Check sheet for the modelled part. Datum: model origin and axes. Units: mm. A direction names the side the tool comes from. Round coordinates to 2 decimals unless told otherwise and drop trailing zeros. Order: outer loops, then holes, each group sorted by start corner. A loop starts at its lowest first (then second) coordinate and runs counter-clockwise, first axis right, second up.
Q1. Depth check by flat-ended pin: P1, Ø3.5, axis at y = 25, z = 10.5, coming from the -X side; P2, Ø0.9, axis at x = 17, y = 19, coming from the -Z side; P3, Ø6, axis at y = 23, z = 10.5, coming from the +X side. Enter the tip coordinate at first touch or a pass-through.
Q2. Cross-section at A-A on x = 2. Record the cut outline in (y, z), then the cut area to 3 significant figures.
Q3. Set-up check for faces 1 (the flat face through (2.935, 17, 16)), 2 (the cylindrical face through (12.252, 20.541, 9.077)), 3 (the flat face through (16, 17, 17.161)), 4 (the flat face through (16.435, 17, 9)), 5 (the flat face through (1.435, 17, 9)): record each of +Z, -Z, +X, -X, +Y, -Y from which the full face is reachable in a straight line by a thin tool's end or side.
Q4. Cross-section at C-C on y = 6.5. Record the cut outline in (x, z).
Q5. Scan lines: probe 1 along Y at (x, z) = (9, 12); probe 2 along Z at (x, y) = (2, 2); probe 3 along Z at (x, y) = (5.25, 18.5). Record each from-to range of solid material in increasing order.
Q6. Cross-section at B-B on z = 11.25. Record the cut outline in (x, y).
Q7. Mould release check, pull along X, two halves, no side actions. Record for faces 6 (the flat face through (-0.065, 17, 18)), 7 (the flat face through (16, 17, 15.161)), 8 (the flat face through (9, 18, 15.161)): +X half, -X half, draft (parallel to the pull), parting line (faces both ways), or undercut.
Q8. Cross-section at D-D on x = 17. Record the cut outline in (y, z), then the cut area to 3 significant figures.
from build123d import *

# Parameters (mm, degrees)
SKETCH1_W           = 6
SKETCH1_H           = 2
BOSS_EXTRUDE1_DEPTH = 35
SKETCH2_R           = 4.5
CUT_EXTRUDE1_DEPTH  = 12


with BuildPart() as part:
    # Sketch1 → Boss-Extrude1 (new body)
    with BuildSketch(Plane(origin=(0, 0, 0), x_dir=(1, 0, 0), z_dir=(0, 1, 0))):
        Polygon((1.435483871, -3.161290323), (1.435483871, -15.161290323), (2.935483871, -15.161290323), (8.935483871, -15.161290323), (8.935483871, -3.161290323), align=None)
        Polygon((16.435483871, -3.161290323), (8.935483871, -3.161290323), (8.935483871, -15.161290323), (14.935483871, -15.161290323), (16.435483871, -15.161290323), align=None)
        with Locations((11.935483871, -16.161290323)):
            Rectangle(SKETCH1_W, SKETCH1_H)
        with Locations((5.935483871, -16.161290323)):
            Rectangle(SKETCH1_W, SKETCH1_H)
        Polygon((8.935483871, -17.161290323), (2.935483871, -17.161290323), (-0.064516129, -17.161290323), (-0.064516129, -19.161290323), (8.935483871, -19.161290323), align=None)
        Polygon((14.935483871, -17.161290323), (8.935483871, -17.161290323), (8.935483871, -19.161290323), (17.935483871, -19.161290323), (17.935483871, -17.161290323), align=None)
    extrude(amount=BOSS_EXTRUDE1_DEPTH)

    # Sketch2 → Cut-Extrude1 (cut)
    with BuildSketch(Plane(origin=(0, 0, 3.161290323), x_dir=(-1, 0, 0), z_dir=(0, 0, -1))):
        with Locations((-8.935483871, 17.5)):
            Circle(SKETCH2_R)
    extrude(amount=-CUT_EXTRUDE1_DEPTH, mode=Mode.SUBTRACT)


solid = part.part
Results found:
1. P1: stops at x = 1.44
1. P2: stops at z = 17.16
1. P3: stops at x = 16.44
2. outline: (0, 3.16) - (35, 3.16) - (35, 15.16) - (0, 15.16) - close; (0, 17.16) - (35, 17.16) - (35, 19.16) - (0, 19.16) - close
2. area: 490 mm2
3. face 1: -X, +Y, -Y
3. face 2: -Z
3. face 3: +X, +Y, -Y
3. face 4: -Z, +X, +Y, -Y
3. face 5: -Z, -X, +Y, -Y
4. outline: (-0.06, 17.16) - (2.94, 17.16) - (2.94, 15.16) - (1.44, 15.16) - (1.44, 3.16) - (16.44, 3.16) - (16.44, 15.16) - (14.94, 15.16) - (14.94, 17.16) - (17.94, 17.16) - (17.94, 19.16) - (-0.06, 19.16) - close
5. probe 1: y = 0 to 13, 22 to 35
5. probe 2: z = 3.16 to 15.16, 17.16 to 19.16
5. probe 3: z = 15.16 to 19.16
6. outline: (1.44, 0) - (16.44, 0) - (16.44, 35) - (1.44, 35) - close; hole circle Ø9 at (8.94, 17.5)
7. face 6: -X half
7. face 7: draft
7. face 8: undercut
8. outline: (0, 17.16) - (35, 17.16) - (35, 19.16) - (0, 19.16) - close
8. area: 70.0 mm2
